Autodesk Fusion 360 part; units mm, degrees
sketch "スケッチ1" plane through (0, 0, 0) normal (0, 0, 1) x (1, 0, 0)
  line L0 (0, 0) -> (72.6, 0)
  line L1 (72.6, 0) -> (72.6, -36.25)
  line L2 (72.6, -36.25) -> (0, -36.25)
  line L3 (0, -36.25) -> (0, 0)
  line L4 (36.3, 0) -> (36.3, -36.25)
  line L5 (0, -18.125) -> (72.6, -18.125)
  line L6 (72.6, -8.625) -> (72.6, -26.625)
  line L7 (58.3, -36.25) -> (14.3, -36.25)
  line L8 (0, -9.125) -> (0, -27.125)
  line L9 (0, -18.125) -> (9.5, -18.125)
  line L10 (0, -9.125) -> (6.4586, -9.125)
  line L11 (0, -27.125) -> (4.6488, -27.125)
  line L12 (6.4586, -9.125) -> (36.3, 0)
  line L13 (14.3, -36.25) -> (12.3, -36.25)
  line L14 (12.3, -36.25) -> (2.2204, -24.2289)
  line L15 (36.3, -18.125) -> (36.3, -32.425)
  line L16 (36.3, -18.125) -> (36.3, -3.825)
  line L17 (66.1414, -9.125) -> (36.3, 0)
  line L18 (60.3, -36.25) -> (70.3796, -24.2289)
  line L19 (58.3, -36.25) -> (60.3, -36.25)
  line L20 (6.4586, -27.125) -> (66.1414, -27.125)
  line L21 (6.4586, -9.125) -> (66.1414, -9.125)
  arc A0 (6.9878, -8.9632) -> (6.4586, -27.125) centre (9.5, -18.125) ccw
  arc A1 (66.1414, -27.125) -> (65.6122, -8.9632) centre (63.1, -18.125) ccw
  circle A2 centre (14.3, -32.425) radius 1.75
  circle A3 centre (36.3, -3.825) radius 1.75
  circle A4 centre (58.3, -32.425) radius 1.75
  circle A5 centre (32.3, -32.425) radius 1
  circle A6 centre (40.3, -32.425) radius 1
  line L22 (36.3, -9.125) -> (36.3, -13.125)
  line L23 (0, -18.125) -> (4, -18.125)
  line L24 (36.3, -13.125) -> (5.4223, -13.125)
  line L25 (36.3, -27.125) -> (36.3, -23.125)
  line L26 (36.3, -23.125) -> (5.4223, -23.125)
  arc A7 (5.4223, -13.125) -> (5.4223, -23.125) centre (13.5, -18.125) ccw
  circle A8 centre (10.55, -18.125) radius 2.55
  circle A9 centre (20.85, -18.125) radius 2.55
  circle A10 centre (31.15, -18.125) radius 2.55
  line L27 (36.3, -13.125) -> (67.1777, -13.125)
  arc A11 (67.1777, -23.125) -> (67.1777, -13.125) centre (59.1, -18.125) ccw
  line L28 (36.3, -23.125) -> (67.1777, -23.125)
  circle A12 centre (41.45, -18.125) radius 2.55
  circle A13 centre (51.75, -18.125) radius 2.55
  circle A14 centre (62.05, -18.125) radius 2.55
  point P0 (36.3, -18.125)
  point P1 (36.3, -3.825)
  point P2 (14.3, -32.425)
  point P3 (58.3, -32.425)
  point P4 (40.3, -32.425)
  point P5 (40.3, -32.425)
  point P6 (32.3, -32.425)
  point P7 (31.15, -18.125)
  point P8 (20.85, -18.125)
  point P9 (10.55, -18.125)
  point P10 (41.45, -18.125)
  point P11 (51.75, -18.125)
  point P12 (62.05, -18.125)
  dimension "d5" = 72.6
  dimension "d6" = 36.25
  dimension "d10" = 44
  dimension "d11" = 9
  dimension "d12" = 18
  dimension "d13" = 9.5
  dimension "d14" = 2
  dimension "d15" = 14.3
  dimension "d16" = 22
  dimension "d17" = 14.3
  dimension "d18" = 3.5
  dimension "d19" = 3.5
  dimension "d20" = 3.5
  dimension "d21" = 4
  dimension "d24" = 2
  dimension "d25" = 2
  dimension "d30" = 4
  dimension "d31" = 4
  dimension "d32" = 9.5
  dimension "d33" = 4
  dimension "d34" = 5.15
  dimension "d35" = 10.3
  dimension "d36" = 10.3
  dimension "d37" = 5.1
  dimension "d38" = 5.1
  dimension "d39" = 5.1
  dimension "d46" = 5.1
  dimension "d47" = 5.1
  dimension "d48" = 5.1
extrude "押し出し1" add sketch "スケッチ1" along normal blind 2 contours L4 L16 L17 L21 A3 | L4 L12 L16 L21 A3 | L4 L5 L9 L16 L21 A0 L22 L23 L24 A7 | L4 L5 L9 L15 L20 A0 L23 L25 L26 A7 | L4 L5 L16 L21 A1 L22 L27 A11 | L4 L5 L9 L16 L24 A7 A8 A9 A10 | L4 L5 L9 L15 L26 A7 A8 A9 A10 | L2 L4 L7 L13 L14 L15 L20 A0 | L4 L5 L15 L20 A1 L25 A11 L28 | L5 L9 A8 | L5 L9 A8 | L4 L5 L16 L27 A11 A12 A13 A14 | L4 L5 L15 A11 L28 A12 A13 A14 | L2 L4 L7 L15 L18 L19 L20 A1 | L5 A14 | L5 A14 | L5 A9 | L5 A9 | L5 A10 | L5 A10 | L5 A12 | L5 A12 | L5 A13 | L5 A13
fillet "フィレット1" radius 1 3 edges at (12.3, -36.25, 1) (60.3, -36.25, 1) (36.3, 0, 1)
sketch "スケッチ2" plane through (0, 0, 2) normal (0, 0, 1) x (-1, 0, 0)
  arc A0 (-36.5924, 0.0894) -> (-36.0076, 0.0894) centre (-36.3, 1.0457) ccw
  line L0 (-36.0076, 0.0894) -> (-6.4586, 9.125)
  arc A1 (-6.4586, 9.125) -> (-2.2204, 24.2289) centre (-9.5, 18.125) ccw
  line L1 (-2.2204, 24.2289) -> (-12.0003, 35.8925)
  arc A2 (-12.0003, 35.8925) -> (-12.7665, 36.25) centre (-12.7665, 35.25) ccw
  line L2 (-12.7665, 36.25) -> (-59.8335, 36.25)
  arc A3 (-59.8335, 36.25) -> (-60.5997, 35.8925) centre (-59.8335, 35.25) ccw
  line L3 (-60.5997, 35.8925) -> (-70.3796, 24.2289)
  arc A4 (-70.3796, 24.2289) -> (-66.1414, 9.125) centre (-63.1, 18.125) ccw
  line L4 (-66.1414, 9.125) -> (-36.5924, 0.0894)
  circle A5 centre (-36.3, 3.825) radius 1.75
  circle A6 centre (-32.3, 32.425) radius 1
  circle A7 centre (-40.3, 32.425) radius 1
  circle A8 centre (-14.3, 32.425) radius 1.75
  circle A9 centre (-58.3, 32.425) radius 1.75
extrude "押し出し2" cut sketch "スケッチ1" along normal blind 2 contours L5 L9 A8 | L5 L9 A8 | L5 A14 | L5 A14 | L5 A9 | L5 A9 | L5 A10 | L5 A10 | L5 A12 | L5 A12 | L5 A13 | L5 A13
Model file for the job. Use its own axes, mm. Give positions to 0.01 mm unless a question says otherwise; leave off trailing zeros. Order: outer loops, then holes, each group sorted by start corner. A loop starts at its lowest first (then second) coordinate and runs counter-clockwise, first axis right, second up. Notation, with made-up numbers: (65.25, 59.25) - (111.25, 59.25) arc R23 ccw to (111.25, 79.25) - close; hole circle Ø9 at (39, 56.25). An arc over 180 degrees is marked (long way). One line per item, written item: value.
Item 1: Slice it at C-C (z = 1.3). Give the number of separate pieces and of enclosed holes in the cut face, then the cut area to 3 significant figures.
Response values:
separate pieces: 1
enclosed holes: 11
area: 1,870 mm2
Item 2: Pin check, flat tip, straight feed: pin 1 Ø1 at (y, z) = (-28, 1) entering from +X. Stop position of the tip, or through.
Response values:
pin 1: x = 67.64
Item 3: Two-plate mould, pull along X, no slides. Class faces 1 (the cylindrical face through (32.08, -31.45, 0.99)), 2 (the flat face through (37, -36.25, 1)), 3 (the flat face through (51.57, -4.67, 0.99)): released by +X, released by -X, zero draft, split by the parting line, or undercut.
Response values:
face 1: undercut
face 2: zero draft
face 3: released by +X
Item 4: Wall check: line 1 (Y direction, x = 40.3, z = 1.4) (3 decimals); line 2 (X direction, y = -33.5, z = 0.2); line 3 (Y direction, x = 20.85, z = 0.55) (3 decimals). Give the ranges that are in metal, low to high.
Response values:
line 1: -36.25 to -33.425, -31.425 to -20.401, -15.849 to -1.223
line 2: 9.99 to 12.92, 15.68 to 56.92, 59.68 to 62.61
line 3: -36.25 to -20.675, -15.575 to -4.724
Item 5: Slice it at B-B (x = 22.5). List the corners of the cut face in (y, z).
Response values:
outline: (-36.25, 0) - (-20.07, 0) - (-20.07, 2) - (-36.25, 2) - close; (-16.18, 0) - (-4.22, 0) - (-4.22, 2) - (-16.18, 2) - close
Item 6: Slice it at D-D (x = 62.05). List the corners of the cut face in (y, z) (3 decimals), then the cut area to 3 significant figures.
Response values:
outline: (-34.163, 0) - (-20.675, 0) - (-20.675, 2) - (-34.163, 2) - close; (-15.575, 0) - (-7.874, 0) - (-7.874, 2) - (-15.575, 2) - close
area: 42.4 mm2
Item 7: Slice it at A-A (x = 40.3). List the corners of the cut face in (y, z) (3 decimals).
Response values:
outline: (-36.25, 0) - (-33.425, 0) - (-33.425, 2) - (-36.25, 2) - close; (-31.425, 0) - (-20.401, 0) - (-20.401, 2) - (-31.425, 2) - close; (-15.849, 0) - (-1.223, 0) - (-1.223, 2) - (-15.849, 2) - close
